Input: part model. Units: mm. Frame: model coordinates. A direction names the side the tool comes from. Give positions to 0.01 mm unless a question says otherwise; leave off trailing zeros. Loops run counter-clockwise (first coordinate to the right, second up) from the corner with the lowest first, then second, coordinate; pieces in that order, holes last.
from build123d import *

# Parameters (mm, degrees)
SKETCH2_R          = 0.8
CUT_EXTRUDE1_DEPTH = 8.4
CUT_EXTRUDE2_DEPTH = 8.4
CIRPATTERN1_COUNT  = 31
CUT_EXTRUDE3_DEPTH = 4.85
CIRPATTERN2_COUNT  = 9
FILLET1_R          = 0.2


with BuildPart() as part:
    # Sketch1 → Revolve1 (revolve)
    with BuildSketch(Plane.XY):
        Polygon((-6.625, 7.4), (-6.625, 4.85), (-2.95, 4.85), (-2.95, 0), (0, 0), (0, 7.4), align=None)
    revolve(axis=Axis((0, 7.4, 0), (0, -1, 0)))

    # Sketch2 → Cut-Extrude1 (cut, through all)
    with BuildSketch(Plane(origin=(0, 7.4, 0), x_dir=(1, 0, 0), z_dir=(0, 1, 0))):
        Circle(SKETCH2_R)
    extrude(amount=-CUT_EXTRUDE1_DEPTH, mode=Mode.SUBTRACT)

    # Sketch4 → Cut-Extrude2 (cut, through all)
    with BuildSketch(Plane(origin=(0, 7.4, 0), x_dir=(1, 0, 0), z_dir=(0, 1, 0))):
        with BuildLine():
            Line((1.333602696, 6.489385861), (0.595196913, 5.853049041))
            Line((0.595196913, 5.853049041), (0, 6.625))
            ThreePointArc((0, 6.625), (0.670240133, 6.591009267), (1.333602696, 6.489385861))
        make_face()
    cut_extrude2 = extrude(amount=-CUT_EXTRUDE2_DEPTH, mode=Mode.SUBTRACT)

    # CirPattern1: Cut-Extrude2 ×31 about axis
    cirpattern1_axis = Axis((0, 0, 0), (0, 1, 0))
    for i in range(1, CIRPATTERN1_COUNT):
        add(cut_extrude2.rotate(cirpattern1_axis, i * 360 / CIRPATTERN1_COUNT), mode=Mode.SUBTRACT)

    # Sketch5 → Cut-Extrude3 (cut)
    with BuildSketch(Plane.XZ):
        with BuildLine():
            Line((0, 2.95), (0.67909598, 1.865800872))
            Line((0.67909598, 1.865800872), (1.896223449, 2.259831107))
            ThreePointArc((1.896223449, 2.259831107), (1.008959423, 2.772093231), (0, 2.95))
        make_face()
    cut_extrude3 = extrude(amount=-CUT_EXTRUDE3_DEPTH, mode=Mode.SUBTRACT)

    # CirPattern2: Cut-Extrude3 ×9 about axis
    cirpattern2_axis = Axis((0, 0, 0), (0, 1, 0))
    for i in range(1, CIRPATTERN2_COUNT):
        add(cut_extrude3.rotate(cirpattern2_axis, i * 360 / CIRPATTERN2_COUNT), mode=Mode.SUBTRACT)

    # Fillet1
    fillet1_edges = [part.edges().sort_by_distance(p)[0] for p in [
        (0, 2.425, 2.95),
        (1.896223449, 2.425, 2.259831107),
        (0.67909598, 2.425, 1.865800872),
        (2.905182871, 2.425, 0.512262124),
        (1.719531385, 2.425, 0.992771908),
        (2.554774941, 2.425, -1.475),
        (1.955378943, 2.425, -0.344786065),
        (1.008959423, 2.425, -2.772093231),
        (-1.008959423, 2.425, -2.772093231),
        (0, 2.425, -1.985543815),
        (-2.554774941, 2.425, -1.475),
        (-1.276282963, 2.425, -1.521014806),
        (-2.905182871, 2.425, 0.512262124),
        (-1.955378943, 2.425, -0.344786065),
        (-1.896223449, 2.425, 2.259831107),
        (-1.719531385, 2.425, 0.992771908),
        (-0.67909598, 2.425, 1.865800872),
    ]]
    fillet(fillet1_edges, radius=FILLET1_R)


solid = part.part
(1) Ray query, probe 1 along Y at (x, z) = (1.25, 5.5); probe 2 along X at (y, z) = (2.5, 0); probe 3 along X at (y, z) = (2.5, 1.75). Return the intervals inside material, ascending.
Values follow:
probe 1: y = 4.85 to 7.4
probe 2: x = -2.34 to -0.8, 0.8 to 2.34
probe 3: x = -1.83 to 1.83
(2) Mould query, pull axis Z, two halves, no side actions, for faces 1 (the flat face through (-2.77, 6.14, 5.6)), 2 (the flat face through (-4.31, 6.143, -4.513)), 3 (the flat face through (-5.477, 6.143, 3.013)). Classes: +Z half, -Z half, draft (parallel to the pull), parting line (faces both ways), or undercut.
Values follow:
face 1: +Z half
face 2: -Z half
face 3: undercut
(3) Reachability of faces 4 (the flat face through (2.761, 6.143, 5.597)), 5 (the flat face through (2.736, 6.143, -5.609)), 6 (the flat face through (-5.114, 6.143, 3.577)) from +Z, -Z, +X, -X, +Y, -Y: full face, straight path, thin tool, end or side. Return the list, or none.
Values follow:
face 4: +Z, +Y, -Y
face 5: -Z, +Y, -Y
face 6: -X, +Y, -Y
(4) Pin query (flat end, axial travel): pin 1 Ø1 at (x, y) = (-5, 5) entering from +Z; pin 2 Ø3 at (y, z) = (3.5, -1.5) entering from -X; pin 3 Ø2 at (x, y) = (3.5, 1.5) entering from +Z. Return the tip coordinate at first contact, or that it passes through.
Values follow:
pin 1: stops at z = 4.06
pin 2: stops at x = -6.55
pin 3: stops at z = 0.68
(5) Cut plane C-C (z = 3.75). Return the cut outline in (x, y).
Values follow:
outline: (-5.16, 4.85) - (5.16, 4.85) - (5.16, 7.4) - (-5.16, 7.4) - close
(6) Cut plane B-B (x = 4). Return the cut outline in (y, z), and give its area (3 significant figures).
Values follow:
outline: (4.85, -4.48) - (7.4, -4.48) - (7.4, 4.96) - (4.85, 4.96) - close
area: 24.1 mm2
(7) Cut plane A-A (z = 0). Return the cut outline in (x, y).
Values follow:
outline: (-6.22, 4.85) - (-2.34, 4.85) - (-2.34, 0) - (-0.8, 0) - (-0.8, 7.4) - (-6.22, 7.4) - close; (0.8, 0) - (2.34, 0) - (2.34, 4.85) - (6.22, 4.85) - (6.22, 7.4) - (0.8, 7.4) - close
